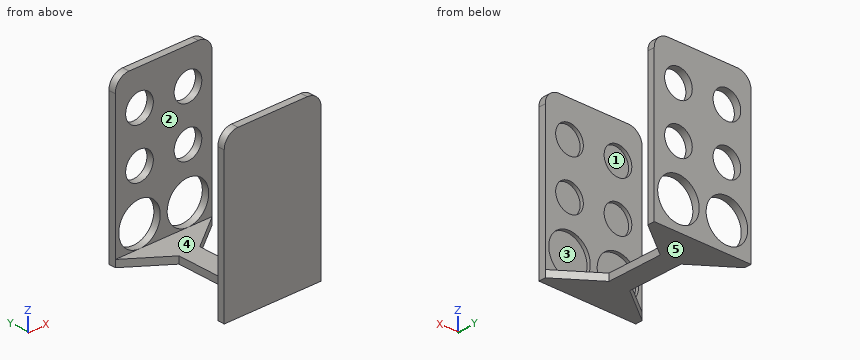
```python
from build123d import *

# Parameters (mm, degrees)
SKETCH1_W               = 139.7
SKETCH1_H               = 6.35
SKETCH1_W_2             = 6.35
SKETCH1_H_2             = 114.3
BOSS_EXTRUDE1_DEPTH     = 88.9
SKETCH2_R               = 19.05
SKETCH2_R_2             = 12.7
CUT_EXTRUDE1_DEPTH      = 111.125
CUT_EXTRUDE3_DEPTH      = 202.205839875
CUT_EXTRUDE3_DEPTH_BACK = 202.205839875
FILLET1_R               = 12.7


with BuildPart() as part:
    # Sketch1 → Boss-Extrude1 (new body)
    with BuildSketch(Plane(origin=(0, 0, 0), x_dir=(0, 0, -1), z_dir=(1, 0, 0))):
        with Locations((-69.85, 111.125)):
            Rectangle(SKETCH1_W, SKETCH1_H)
        with Locations((3.175, 57.15)):
            Rectangle(SKETCH1_W_2, SKETCH1_H_2)
        with Locations((-69.85, 3.175)):
            Rectangle(SKETCH1_W, SKETCH1_H)
    extrude(amount=BOSS_EXTRUDE1_DEPTH)

    # Sketch2 → Cut-Extrude1 (cut)
    with BuildSketch(Plane(origin=(0, 114.3, 0), x_dir=(1, 0, 0), z_dir=(0, 1, 0))):
        with Locations(Location((66.675, -19.05, 0), (0, 0, 270))):
            Circle(SKETCH2_R)
        with Locations(Location((66.675, -63.5, 0), (0, 0, 270))):
            Circle(SKETCH2_R_2)
        with Locations(Location((66.675, -107.95, 0), (0, 0, 270))):
            Circle(SKETCH2_R_2)
        with Locations(Location((22.225, -107.95, 0), (0, 0, 270))):
            Circle(SKETCH2_R_2)
        with Locations(Location((22.225, -63.5, 0), (0, 0, 270))):
            Circle(SKETCH2_R_2)
        with Locations(Location((22.225, -19.05, 0), (0, 0, 270))):
            Circle(SKETCH2_R)
    extrude(amount=-CUT_EXTRUDE1_DEPTH, mode=Mode.SUBTRACT)

    # Sketch4 → Cut-Extrude3 (cut, two sides: drawn at the far end of the back side and taken through both)
    with BuildSketch(Plane.XY.offset(-CUT_EXTRUDE3_DEPTH_BACK)):
        Polygon((34.925, 31.75), (34.925, 82.55), (0, 107.95), (0, 6.35), align=None)
        Polygon((53.975, 82.55), (53.975, 31.75), (88.9, 6.35), (88.9, 107.95), align=None)
    extrude(amount=CUT_EXTRUDE3_DEPTH + CUT_EXTRUDE3_DEPTH_BACK, mode=Mode.SUBTRACT)

    # Fillet1
    fillet1_edges = [part.edges().sort_by_distance(p)[0] for p in [
        (88.9, 111.125, 139.7),
        (0, 3.175, 139.7),
        (0, 111.125, 139.7),
        (88.9, 3.175, 139.7),
    ]]
    fillet(fillet1_edges, radius=FILLET1_R)


solid = part.part
```
Verification items for the finished model (mm, model axes). Face numbers are marked on the shaded views. A direction names the side the tool comes from. Round coordinates to 2 decimals unless told otherwise and drop trailing zeros. Write each loop counter-clockwise with the first axis right and the second up, starting at its lowest first coordinate (ties: lowest second). Pieces come first, ordered by that corner, then holes. Notation, with made-up numbers: (35, -31.5) -> (81, -31.5) arc R18 ccw to (81, -16.5) -> close; hole circle Ø4 at (42, 75). An arc over 180 degrees is marked (long way). Write each question's results on one line, items separated by ' | '. Start each with the question number.
1. Cross-section at C-C (x = 6). Enter the section's corners in (y, z) (3 decimals).
2. Cross-section at B-B (z = 19.05). Enter the section's corners in (x, y) (3 decimals).
3. Depth check by flat-ended pin: P1, Ø23, axis at x = 22.225, z = 107.95, coming from the +Y side (3 decimals); P2, Ø1.9, axis at y = 65.5, z = -4.5, coming from the -X side (3 decimals). Enter the tip coordinate at first touch or a pass-through.
4. Material ranges on probe 1 along X at (y, z) = (4.65, 63.5) (3 decimals); probe 2 along X at (y, z) = (5.3, 19.05) (3 decimals); probe 3 along Y at (x, z) = (46, 128), recorded low to high. Write a range as from..to.
5. Set-up check for the marked faces 3, 4 and 5: record each of +Z, -Z, +X, -X, +Y, -Y from which the full face is reachable in a straight line by a thin tool's end or side.
6. Draft check along X on the marked faces 1 and 2. Enter one of: +X half, -X half, draft (parallel to the pull), parting line (faces both ways), or undercut.
7. Cross-section at A-A (z = 81.5). Enter the section's corners in (x, y), then the cut area to 3 significant figures.
8. Cross-section at D-D (x = 39.5). Enter the section's corners in (y, z) (3 decimals), then the cut area to 3 significant figures.
Solutions:
1) outline: (0, -6.35) -> (10.714, -6.35) -> (10.714, 0) -> (6.35, 0) -> (6.35, 9.067) -> (3.175, 9.067) -> (3.175, 29.033) -> (6.35, 29.033) -> (6.35, 137.789) -> (0, 137.789) -> close; (103.586, -6.35) -> (114.3, -6.35) -> (114.3, 9.067) -> (107.95, 9.067) -> (107.95, 0) -> (103.586, 0) -> close; (107.95, 29.033) -> (114.3, 29.033) -> (114.3, 137.789) -> (107.95, 137.789) -> close
2) outline: (0, 0) -> (88.9, 0) -> (88.9, 6.35) -> (85.725, 6.35) -> (85.725, 3.175) -> (47.625, 3.175) -> (47.625, 6.35) -> (41.275, 6.35) -> (41.275, 3.175) -> (3.175, 3.175) -> (3.175, 6.35) -> (0, 6.35) -> close; (0, 107.95) -> (3.175, 107.95) -> (3.175, 114.3) -> (0, 114.3) -> close; (41.275, 107.95) -> (47.625, 107.95) -> (47.625, 114.3) -> (41.275, 114.3) -> close; (85.725, 107.95) -> (88.9, 107.95) -> (88.9, 114.3) -> (85.725, 114.3) -> close
3) P1: stops at y = 3.175 | P2: stops at x = 34.925
4) probe 1: x = 0..9.525, 34.925..53.975, 79.375..88.9 | probe 2: x = 0..3.175, 41.275..47.625, 85.725..88.9 | probe 3: y = 0..6.35, 107.95..114.3
5) face 3: +Y | face 4: +Z, +X, -X | face 5: -Z, +X, -X, +Y, -Y
6) face 1: undercut | face 2: draft
7) outline: (0, 0) -> (88.9, 0) -> (88.9, 6.35) -> (0, 6.35) -> close; (0, 107.95) -> (88.9, 107.95) -> (88.9, 114.3) -> (0, 114.3) -> close | area: 1,130 mm2
8) outline: (0, -6.35) -> (114.3, -6.35) -> (114.3, 11.02) -> (107.95, 11.02) -> (107.95, 0) -> (6.35, 0) -> (6.35, 11.02) -> (3.175, 11.02) -> (3.175, 27.08) -> (6.35, 27.08) -> (6.35, 139.7) -> (0, 139.7) -> close; (107.95, 27.08) -> (114.3, 27.08) -> (114.3, 139.7) -> (107.95, 139.7) -> close | area: 2,350 mm2
